Can you work these out from the model? Positions are in its coordinate system, mm. Face numbers are marked on the shaded views. A direction names the side the tool comes from. Give positions to 0.01 mm unless a question says otherwise; leave off trailing zeros. Order: outer loops, then holes, each group sorted by start corner. A loop starts at its lowest first (then second) coordinate and runs counter-clockwise, first axis right, second up. Notation, with made-up numbers: M 47.5,89.5 L 98.5,89.5 A19 cw 98.5,102.5 Z; hole C -8.75,-3 d4. An arc over 180 degrees is marked long. One line per question, with ' | ' between items. Start each with the question number.
1) Please list where these lines run through material, in increasing order: line 1 along Z through (x, y) = (-38.5, 6.25) (3 decimals); line 2 along Y through (x, z) = (-52, -28) (3 decimals). Write a range as [from, to].
2) For the marked faces 1 and 2, which set-ups out of +Z, -Z, +X, -X, +Y, -Y let a thin tool reach every point of the face, with its end or its side?
3) If we section it at B-B, the plane z = -94: Please give me the cut outline in (x, y) (3 decimals).
4) If we section it at A-A, the plane y = 2: Please give me the cut outline in (x, z) (3 decimals).
5) I'm going to push flat-ended pins straight in: pin 1 Ø1.5 at (y, z) = (10.5, -58.5) entering from -X (3 decimals); pin 2 Ø1.5 at (x, z) = (-16, -42) entering from +Y (3 decimals); pin 3 Ø8 at (x, y) = (-17, 3.5) entering from -Z. Where does each tip first touch, or does it pass through?
6) If we section it at C-C, the plane x = -57.5: Please give me the cut outline in (y, z) (3 decimals), plus the area to 3 significant figures.
Autodesk Inventor part; units mm, degrees
ref_plane "YZ Plane" through (0, 0, 0) normal (1, 0, 0) x (0, 1, 0)
ref_plane "XZ Plane" through (0, 0, 0) normal (0, 1, 0) x (-1, 0, 0)
ref_plane "XY Plane" through (0, 0, 0) normal (0, 0, 1) x (1, 0, 0)
sketch "Sketch1" plane through (0, 0, 0) normal (0, 1, 0) x (-1, 0, 0)
  line L0 (0, 0) -> (101.6, 0)
  line L1 (101.6, 0) -> (101.6, -3.175)
  line L2 (101.6, -3.175) -> (3.175, -3.175)
  line L3 (0, -3.175) -> (0, 0)
  line L4 (0, 0) -> (3.175, 0)
  line L5 (3.175, -3.175) -> (3.175, -101.6)
  line L6 (3.175, -101.6) -> (0, -101.6)
  line L7 (0, -101.6) -> (0, 0)
  dimension "d0" = 101.6
  dimension "d1" = 3.175
  dimension "d2" = 3.175
  dimension "d3" = 101.6
extrude "Extrusion1" add sketch "Sketch1" along normal blind 28.575
sketch "Sketch2" plane through (0, 0, 0) normal (0, -1, 0) x (1, 0, 0)
  line L0 (-3.175, -101.6) -> (-3.175, -3.175)
  line L1 (-3.175, -3.175) -> (-101.6, -3.175)
  line L2 (-3.175, -101.6) -> (-101.6, -3.175)
  point P0 (0, 0)
extrude "Extrusion2" add sketch "Sketch2" against normal blind 3.175
properties part number "Right Angle Gig"
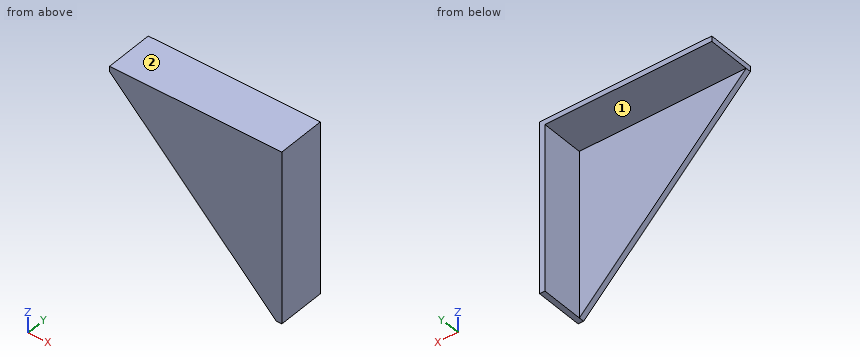
Results found:
1) line 1: z = [-3.175, 0] | line 2: y = [0, 3.175]
2) face 1: -Z, -X, +Y | face 2: +Z, +X, -X, +Y, -Y
3) outline: M -10.775,0 L 0,0 L 0,28.575 L -3.175,28.575 L -3.175,3.175 L -10.775,3.175 Z
4) outline: M -101.6,-3.175 L -3.175,-101.6 L 0,-101.6 L 0,0 L -101.6,0 Z
5) pin 1: stops at x = -3.175 | pin 2: stops at y = 3.175 | pin 3: stops at z = -91.76
6) outline: M 0,-47.275 L 3.175,-47.275 L 3.175,-3.175 L 28.575,-3.175 L 28.575,0 L 0,0 Z | area: 231 mm²
